Check sheet for the modelled part. Datum: model origin and axes. Units: mm. A direction names the side the tool comes from. Give positions to 0.01 mm unless a question says otherwise; leave off trailing zeros. Loops run counter-clockwise (first coordinate to the right, second up) from the corner with the lowest first, then second, coordinate; pieces in that order, holes last. Notation, with made-up numbers: (-29.5, 63.5) -> (16.5, 63.5) arc R24 ccw to (16.5, 83.5) -> close; hole circle Ø1 at (38.25, 52.25). An arc over 180 degrees is marked (long way). Answer as CSV lines item,"result". Start each with the question number.
(1) Access from +Z, -Z, +X, -X, +Y, -Y to the whole of each face (thin tool, end or side, straight path). Record for faces 4 (the face through (-32.369, 32.528, 11.27)), 5 (the face through (31.24, -31.117, 12.558)), 6 (the face through (-38.1, 0, 11)), 7 (the face through (-32.528, -32.369, 11.27)).
(2) Release check for a two-part mould opening along Z. For faces 1 (the face through (8, 1, 0)), 2 (the face through (-2.123, 0, 1)), 3 (the face through (35.56, 0, 13)) record: pulls with the +Z half, pulls with the -Z half, needs draft (parallel to the pull), parting line crosses it, or undercut.
(3) Section check A-A on z = 9.5. Enter the section's corners in (x, y), plus the area to 3 significant figures.
(4) Material ranges on line 1 (Y direction, x = 3, z = 15); line 2 (Z direction, x = -17.5, y = -35), recorded low to high. Write a range as from..to.
(5) Gauge pin test, flat ends, axial feed: pin 1 Ø1.5 at (x, y) = (13.5, -9.5) entering from -Z; pin 2 Ø1.5 at (x, z) = (27.5, 8) entering from -Y; pin 3 Ø5 at (y, z) = (8, 13.5) entering from -X; pin 4 Ø2 at (y, z) = (28.5, 5) entering from -X. Record the tip position at first contact, or that the pin passes through.
from build123d import *

# Parameters (mm, degrees)
F3_DEPTH = 2.54
F3_TAPER = -3
F0_W     = 2.54
F0_H     = 53.594
F0_W_2   = 53.594
F0_H_2   = 2.54
F4_DEPTH = 25.4
F0_H_3   = 8.763
F0_W_3   = 8.763
F2_W     = 53.594
F2_H     = 53.594
F2_W_2   = 4.2453631759
F2_H_2   = 20.1131701469
F6_DEPTH = 2.54


with BuildPart() as f3:
    # F5 (on offset) → F3 (new body)
    with BuildSketch(Plane.XY.offset(22.86)):
        Polygon((-26.797, -26.797), (-38.1, -26.797), (-26.797, -38.1), align=None)
        with BuildLine():
            ThreePointArc((-18.0581535106, -26.797), (-22.8492463466, -22.8492463466), (-26.797, -18.0581535106))
            Line((-26.797, -18.0581535106), (-26.797, -26.797))
            Line((-26.797, -26.797), (-18.0581535106, -26.797))
        make_face()
        Polygon((38.1, 26.797), (26.797, 38.1), (26.797, 26.797), align=None)
        with BuildLine():
            Line((26.797, 18.0581535106), (26.797, 26.797))
            Line((26.797, 26.797), (18.0581535106, 26.797))
            ThreePointArc((18.0581535106, 26.797), (22.8492463466, 22.8492463466), (26.797, 18.0581535106))
        make_face()
        with BuildLine():
            Line((-18.0581535106, 26.797), (-26.797, 26.797))
            Line((-26.797, 26.797), (-26.797, 18.0581535106))
            ThreePointArc((-26.797, 18.0581535106), (-22.8492463466, 22.8492463466), (-18.0581535106, 26.797))
        make_face()
        Polygon((26.797, -38.1), (38.1, -26.797), (26.797, -26.797), align=None)
        with BuildLine():
            Line((38.1, 26.797), (26.797, 26.797))
            Line((26.797, 26.797), (26.797, 18.0581535106))
            ThreePointArc((26.797, 18.0581535106), (30.9037757664, 9.4410148075), (32.3137140733, 0))
            ThreePointArc((32.3137140733, 0), (30.9037757664, -9.4410148075), (26.797, -18.0581535106))
            Line((26.797, -18.0581535106), (26.797, -26.797))
            Line((26.797, -26.797), (38.1, -26.797))
            Line((38.1, -26.797), (38.1, 26.797))
        make_face()
        with BuildLine():
            Line((26.797, -38.1), (26.797, -26.797))
            Line((26.797, -26.797), (18.0581535106, -26.797))
            ThreePointArc((18.0581535106, -26.797), (0, -32.3137140733), (-18.0581535106, -26.797))
            Line((-18.0581535106, -26.797), (-26.797, -26.797))
            Line((-26.797, -26.797), (-26.797, -38.1))
            Line((-26.797, -38.1), (26.797, -38.1))
        make_face()
        Polygon((-26.797, 26.797), (-26.797, 38.1), (-38.1, 26.797), align=None)
        with BuildLine():
            Line((26.797, 26.797), (26.797, 38.1))
            Line((26.797, 38.1), (-26.797, 38.1))
            Line((-26.797, 38.1), (-26.797, 26.797))
            Line((-26.797, 26.797), (-18.0581535106, 26.797))
            ThreePointArc((-18.0581535106, 26.797), (0, 32.3137140733), (18.0581535106, 26.797))
            Line((18.0581535106, 26.797), (26.797, 26.797))
        make_face()
        with BuildLine():
            Line((26.797, -26.797), (26.797, -18.0581535106))
            ThreePointArc((26.797, -18.0581535106), (22.8492463466, -22.8492463466), (18.0581535106, -26.797))
            Line((18.0581535106, -26.797), (26.797, -26.797))
        make_face()
        with BuildLine():
            Line((-26.797, 18.0581535106), (-26.797, 26.797))
            Line((-26.797, 26.797), (-38.1, 26.797))
            Line((-38.1, 26.797), (-38.1, -26.797))
            Line((-38.1, -26.797), (-26.797, -26.797))
            Line((-26.797, -26.797), (-26.797, -18.0581535106))
            ThreePointArc((-26.797, -18.0581535106), (-32.3137140733, 0), (-26.797, 18.0581535106))
        make_face()
    extrude(amount=F3_DEPTH, taper=F3_TAPER)

    # F0 (on Top) → F4 (join)
    with BuildSketch(Plane.XY):
        with Locations((36.83, 0)):
            Rectangle(F0_W, F0_H)
        Polygon((26.797, -38.1), (38.1, -26.797), (35.56, -26.797), (26.797, -35.56), align=None)
        with Locations((0, -36.83)):
            Rectangle(F0_W_2, F0_H_2)
        Polygon((-35.56, -26.797), (-38.1, -26.797), (-26.797, -38.1), (-26.797, -35.56), align=None)
        with Locations((-36.83, 0)):
            Rectangle(F0_W, F0_H)
        Polygon((-26.797, 35.56), (-26.797, 38.1), (-38.1, 26.797), (-35.56, 26.797), align=None)
        with Locations((0, 36.83)):
            Rectangle(F0_W_2, F0_H_2)
        Polygon((38.1, 26.797), (26.797, 38.1), (26.797, 35.56), (35.56, 26.797), align=None)
    extrude(amount=F4_DEPTH)

    # F0 (on Top) + F2 (on face) → F6 (join)
    with BuildSketch(Plane.XY):
        Polygon((35.56, 26.797), (26.797, 35.56), (26.797, 26.797), align=None)
        with Locations((0, 31.1785)):
            Rectangle(F0_W_2, F0_H_3)
        with Locations((31.1785, 0)):
            Rectangle(F0_W_3, F0_H)
        Polygon((-26.797, 26.797), (-26.797, 35.56), (-35.56, 26.797), align=None)
        with Locations((-31.1785, 0)):
            Rectangle(F0_W_3, F0_H)
        Polygon((-26.797, -35.56), (-26.797, -26.797), (-35.56, -26.797), align=None)
        with Locations((0, -31.1785)):
            Rectangle(F0_W_2, F0_H_3)
        Polygon((35.56, -26.797), (26.797, -26.797), (26.797, -35.56), align=None)
    with BuildSketch(Plane.XY):
        Rectangle(F2_W, F2_H)
        Rectangle(F2_W_2, F2_H_2, mode=Mode.SUBTRACT)
    extrude(amount=F6_DEPTH)


solid = f3.part
Working result:
1,face 4,"-Z, -X, +Y"
1,face 5,"none"
1,face 6,"-Z, -X, +Y, -Y"
1,face 7,"-Z, -X, -Y"
2,face 1,"pulls with the -Z half"
2,face 2,"needs draft"
2,face 3,"undercut"
3,outline,"(-38.1, -26.8) -> (-26.8, -38.1) -> (26.8, -38.1) -> (38.1, -26.8) -> (38.1, 26.8) -> (26.8, 38.1) -> (-26.8, 38.1) -> (-38.1, 26.8) -> close; hole (-35.56, -26.8) -> (-26.8, -35.56) -> (26.8, -35.56) -> (35.56, -26.8) -> (35.56, 26.8) -> (26.8, 35.56) -> (-26.8, 35.56) -> (-35.56, 26.8) -> close"
3,area,"646 mm^2"
4,line 1,"y = -38.1..-35.56, 35.56..38.1"
4,line 2,"z = 0..2.54, 22.86..25.4"
5,pin 1,"stops at z = 0"
5,pin 2,"stops at y = -38.1"
5,pin 3,"stops at x = -38.1"
5,pin 4,"stops at x = -37.4"
